Autodesk Inventor part; units mm, degrees
ref_plane "YZ Plane" through (0, 0, 0) normal (1, 0, 0) x (0, 1, 0)
ref_plane "XZ Plane" through (0, 0, 0) normal (0, 1, 0) x (-1, 0, 0)
ref_plane "XY Plane" through (0, 0, 0) normal (0, 0, 1) x (1, 0, 0)
sketch "Sketch5" plane through (0, 0, 0) normal (0, 0, 1) x (1, 0, 0)
  line L0 (-15, 15) -> (15, 15) construction
  line L1 (15, 15) -> (15, -15) construction
  line L2 (15, -15) -> (-15, -15) construction
  line L3 (-15, -15) -> (-15, 15) construction
  line L4 (-15, 15) -> (15, -15) construction
  line L5 (15, 15) -> (-15, -15) construction
  circle A0 centre (-15, 15) radius 2
  circle A1 centre (15, 15) radius 2
  circle A2 centre (15, -15) radius 2
  circle A3 centre (-15, -15) radius 2
  line L6 (-15, 20) -> (15, 20)
  line L7 (20, 15) -> (20, -15)
  line L8 (15, -20) -> (-15, -20)
  line L9 (-20, -15) -> (-20, 15)
  line L10 (-20, 20) -> (20, -20) construction
  line L11 (20, 20) -> (-20, -20) construction
  arc A4 (20, 15) -> (15, 20) centre (15, 15) ccw
  arc A5 (15, -20) -> (20, -15) centre (15, -15) ccw
  arc A6 (-20, -15) -> (-15, -20) centre (-15, -15) ccw
  arc A7 (-15, 20) -> (-20, 15) centre (-15, 15) ccw
  point P0 (0, 0)
  dimension "d16" = 4
  dimension "d17" = 30
  dimension "d18" = 40
  dimension "d20" = 5
extrude "Extrusion5" add sketch "Sketch5" along normal blind 5
sketch "Sketch6" plane through (0, 0, 5) normal (0, 0, 1) x (1, 0, 0)
  line L0 (-15, -20) -> (15, -20)
  line L1 (-6, 20) -> (6, 20)
  line L2 (6, 20) -> (6, -20)
  line L3 (6, -20) -> (-6, -20)
  line L4 (-6, -20) -> (-6, 20)
  line L5 (-6, 20) -> (6, -20) construction
  line L6 (6, 20) -> (-6, -20) construction
  point P0 (0, 0)
  dimension "d23" = 12
extrude "Extrusion6" add sketch "Sketch6" along normal blind 40
fillet "Fillet2" radius 5 2 edges at (6, 0, 5) (-6, 0, 5)
sketch "Sketch7" plane through (6, -20, 45) normal (1, 0, 0) x (0, 0, -1)
  circle A0 centre (20, 20) radius 8.5
  circle A1 centre (20, 20) radius 20
  line L0 (0, 0) -> (0, 40)
  line L1 (40, 0) -> (40, 40)
  line L2 (35, 0) -> (0, 0)
  line L3 (20, 0) -> (0, 0)
  line L4 (0, 0) -> (0, 40)
  line L5 (0, 40) -> (20, 40)
  line L6 (35, 40) -> (0, 40)
  point P0 (45, 20)
  point P1 (0, 20)
  dimension "d27" = 17
extrude "Extrusion7" cut sketch "Sketch7" against normal blind 50 contours A0 | A1 L0 L5 | L2 L0 A1
sketch "Sketch1" plane through (0, 0, 0) normal (0, 1, 0) x (-1, 0, 0)
  line L0 (27.5, 22.5) -> (-27.5, 22.5)
  line L1 (-27.5, 22.5) -> (-27.5, -22.5)
  line L2 (-27.5, -22.5) -> (27.5, -22.5)
  line L3 (27.5, -22.5) -> (27.5, 22.5)
  point P0 (0, 0)
  point P1 (27.5, 0)
  point P2 (0, -22.5)
  dimension "d0" = 45
  dimension "d1" = 55
sketch "Sketch2" plane through (0, 10, 0) normal (0, 1, 0) x (1, 0, 0)
  line L0 (-27.5, 22.5) -> (-27.5, -22.5)
  line L1 (-27.5, -22.5) -> (27.5, -22.5)
  line L2 (-27.5, 22.5) -> (-19.5, 22.5)
  line L3 (-19.5, 22.5) -> (-19.5, -22.5)
  line L4 (-19.5, -22.5) -> (-27.5, -22.5)
  line L5 (-27.5, -22.5) -> (-27.5, 22.5)
  line L6 (27.5, -22.5) -> (27.5, 22.5)
  line L7 (27.5, 22.5) -> (19.5, 22.5)
  line L8 (19.5, 22.5) -> (19.5, -22.5)
  line L9 (19.5, -22.5) -> (27.5, -22.5)
  line L10 (27.5, -22.5) -> (27.5, 22.5)
  point P0 (0, 0)
  dimension "d4" = 8
  dimension "d5" = 8
sketch "Sketch4" plane through (0, 0, 0) normal (0, -1, 0) x (1, 0, 0)
  line L0 (15, 15) -> (-15, 15) construction
  line L1 (-15, 15) -> (-15, -15) construction
  line L2 (-15, -15) -> (15, -15) construction
  line L3 (15, -15) -> (15, 15) construction
  line L4 (15, 15) -> (-15, -15) construction
  line L5 (-15, 15) -> (15, -15) construction
  circle A0 centre (15, -15) radius 2
  circle A1 centre (-15, -15) radius 2
  circle A2 centre (-15, 15) radius 2
  circle A3 centre (15, 15) radius 2
  point P0 (0, 0)
  dimension "d12" = 30
  dimension "d13" = 4
sketch "Sketch3" plane through (27.5, 0, 22.5) normal (1, 0, 0) x (0, 0, -1)
  circle A0 centre (22.5, 25) radius 15
  line L0 (22.5, 25) -> (22.5, 47.5) construction
  line L1 (45, 47.5) -> (0, 47.5)
  line L2 (22.5, 25) -> (45, 25) construction
  line L3 (45, 0) -> (45, 47.5)
  point P0 (22.5, 0)
  dimension "d9" = 30
properties part number "Hinge"
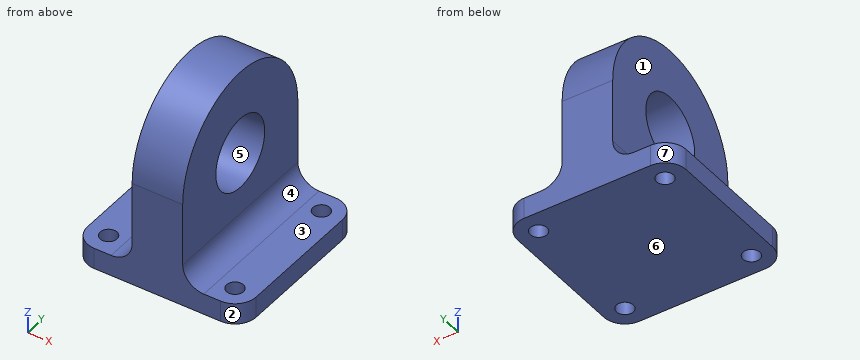
Input: part model. Units: mm. Frame: model coordinates. Face numbers are marked on the shaded views. A direction names the side the tool comes from. Give positions to 0.01 mm unless a question says otherwise; leave off trailing zeros. Loops run counter-clockwise (first coordinate to the right, second up) from the corner with the lowest first, then second, coordinate; pieces in that order, holes last. Notation, with made-up numbers: (-36.75, -4) -> (8.25, -4) arc R23 ccw to (8.25, 8) -> close; hole circle Ø3 at (8.25, -29.5). An arc over 180 degrees is marked (long way). Use a Markdown table: item, result.
Q1. Section query C-C, the plane z = 32. Return the cut outline in (x, y) (3 decimals), plus the area to 3 significant figures.
Entries:
| item | result |
|---|---|
| outline | (-6, -18.735) -> (6, -18.735) -> (6, -4.822) -> (-6, -4.822) -> close; (-6, 4.822) -> (6, 4.822) -> (6, 18.735) -> (-6, 18.735) -> close |
| area | 334 mm² |
Q2. Pull-direction query (Z, two-part tool) for the marked faces 4, 5, 6 and 7; classes: pulls with the +Z half, pulls with the -Z half, needs draft (parallel to the pull), parting line crosses it, or undercut.
Entries:
| item | result |
|---|---|
| face 4 | pulls with the +Z half |
| face 5 | undercut |
| face 6 | pulls with the -Z half |
| face 7 | needs draft |
Q3. Section query D-D, the plane z = 37. Return the cut outline in (x, y), plus the area to 3 significant figures.
Entries:
| item | result |
|---|---|
| outline | (-6, -16) -> (6, -16) -> (6, 16) -> (-6, 16) -> close |
| area | 384 mm² |
Q4. Access query for the marked faces 1, 2 and 3. Directions: +Z, -Z, +X, -X, +Y, -Y. A direction counts if a zero-diameter tool reaches every point of the face in a straight line with its end or side. Return the directions, or none.
Entries:
| item | result |
|---|---|
| face 1 | +Z, -X, +Y, -Y |
| face 2 | +Z, -Z, +X, -Y |
| face 3 | +Z, +X, +Y, -Y |
Q5. Section query B-B, the plane z = 23. Return the cut outline in (x, y).
Entries:
| item | result |
|---|---|
| outline | (-6, -20) -> (6, -20) -> (6, -8.26) -> (-6, -8.26) -> close; (-6, 8.26) -> (6, 8.26) -> (6, 20) -> (-6, 20) -> close |
Q6. Section query A-A, the plane y = 0. Return the cut outline in (x, z), plus the area to 3 significant figures.
Entries:
| item | result |
|---|---|
| outline | (-20, 0) -> (20, 0) -> (20, 5) -> (11, 5) arc R5 cw to (6, 10) -> (6, 16.5) -> (-6, 16.5) -> (-6, 10) arc R5 cw to (-11, 5) -> (-20, 5) -> close; (-6, 33.5) -> (6, 33.5) -> (6, 45) -> (-6, 45) -> close |
| area | 487 mm² |
Q7. Ray query, probe 1 along Y at (x, z) = (-15, 3.45); probe 2 along X at (y, z) = (10, 16); probe 3 along Z at (x, y) = (12, 9). Return the intervals inside material, ascending. Write a range as from..to.
Entries:
| item | result |
|---|---|
| probe 1 | y = -20..-17, -13..13, 17..20 |
| probe 2 | x = -6..6 |
| probe 3 | z = 0..5 |
Q8. First-contact query: P1, Ø5, axis at y = 2.5, z = 22, coming from the +X side; P2, Ø6.5, axis at x = 15, y = 15, coming from the +Z side; P3, Ø12, axis at x = -6, y = 3, coming from the +Z side; P4, Ø17.5, axis at y = -2, z = 25, coming from the -X side. Flat tips, straight axial feed; report the tip coordinate or a pass-through.
Entries:
| item | result |
|---|---|
| P1 | passes through |
| P2 | stops at z = 5 |
| P3 | stops at z = 45 |
| P4 | stops at x = -6 |
